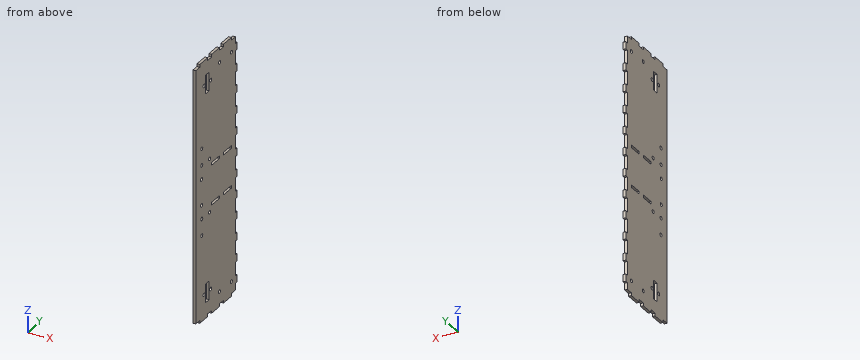
from build123d import *

# Parameters (mm, degrees)
SKETCH1_W               = 279.4
SKETCH1_H               = 76.2
BOSS_EXTRUDE1_DEPTH     = 3
SKETCH3_W               = 3
SKETCH3_H               = 7.8
CUT_EXTRUDE1_DEPTH      = 145.833352512
LPATTERN1_COUNT         = 4
LPATTERN1_PITCH         = 22.8
MIRROR1_COPY_1_SKETCH_W = 3
MIRROR1_COPY_1_SKETCH_H = 7.8
MIRROR1_COPY_1_DEPTH    = 145.833352512
MIRROR1_COPY_2_SKETCH_W = 3
MIRROR1_COPY_2_SKETCH_H = 7.8
MIRROR1_COPY_2_DEPTH    = 145.833352512
MIRROR1_COPY_3_SKETCH_W = 3
MIRROR1_COPY_3_SKETCH_H = 7.8
MIRROR1_COPY_3_DEPTH    = 145.833352512
SKETCH5_W               = 3
SKETCH5_H               = 15
CUT_EXTRUDE3_DEPTH      = 10
SKETCH9_W               = 3
SKETCH9_H               = 7.8
BOSS_EXTRUDE2_DEPTH     = 3
LPATTERN4_COUNT         = 12
LPATTERN4_PITCH         = 22.8
LPATTERN5_COUNT         = 2
LPATTERN5_PITCH         = 22.8
MIRROR2_COPY_1_SKETCH_W = 3
MIRROR2_COPY_1_SKETCH_H = 15
MIRROR2_COPY_1_DEPTH    = 10
F_6_CLEARANCE_HOLE1_D   = 3.7973
CUT_EXTRUDE4_REACH      = 147.651
SKETCH12_W              = 20.2
SKETCH12_H              = 6.7
F_6_CLEARANCE_HOLE2_D   = 3.7973
F_6_CLEARANCE_HOLE3_D   = 3.7973
F_6_CLEARANCE_HOLE4_D   = 3.7973


with BuildPart() as part:
    # Sketch1 → Boss-Extrude1 (new body)
    with BuildSketch(Plane(origin=(0, 0, 0), x_dir=(0, 0, -1), z_dir=(1, 0, 0))):
        Rectangle(SKETCH1_W, SKETCH1_H)
    extrude(amount=-BOSS_EXTRUDE1_DEPTH)

    # Sketch3 → Cut-Extrude1 (cut, through all)
    with BuildSketch(Plane.ZY.offset(3)):
        with Locations((-138.2, 34.2)):
            Rectangle(SKETCH3_W, SKETCH3_H)
    cut_extrude1 = extrude(amount=-CUT_EXTRUDE1_DEPTH, mode=Mode.SUBTRACT)

    # LPattern1: Cut-Extrude1 ×4
    with Locations(*[(0, -i * LPATTERN1_PITCH, 0) for i in range(1, LPATTERN1_COUNT)]):
        add(cut_extrude1, mode=Mode.SUBTRACT)

    # Mirror1: Cut-Extrude1 across plane
    add(cut_extrude1.mirror(Plane.XY), mode=Mode.SUBTRACT)

    # Mirror1 copy 1 sketch → Mirror1 copy 1 (cut, through all)
    with BuildSketch(Plane(origin=(-3, -22.8, 0), x_dir=(0, 0, -1), z_dir=(-1, 0, 0))):
        with Locations((-138.2, -34.2)):
            Rectangle(MIRROR1_COPY_1_SKETCH_W, MIRROR1_COPY_1_SKETCH_H)
    extrude(amount=-MIRROR1_COPY_1_DEPTH, mode=Mode.SUBTRACT)

    # Mirror1 copy 2 sketch → Mirror1 copy 2 (cut, through all)
    with BuildSketch(Plane(origin=(-3, -45.6, 0), x_dir=(0, 0, -1), z_dir=(-1, 0, 0))):
        with Locations((-138.2, -34.2)):
            Rectangle(MIRROR1_COPY_2_SKETCH_W, MIRROR1_COPY_2_SKETCH_H)
    extrude(amount=-MIRROR1_COPY_2_DEPTH, mode=Mode.SUBTRACT)

    # Mirror1 copy 3 sketch → Mirror1 copy 3 (cut, through all)
    with BuildSketch(Plane(origin=(-3, -68.4, 0), x_dir=(0, 0, -1), z_dir=(-1, 0, 0))):
        with Locations((-138.2, -34.2)):
            Rectangle(MIRROR1_COPY_3_SKETCH_W, MIRROR1_COPY_3_SKETCH_H)
    extrude(amount=-MIRROR1_COPY_3_DEPTH, mode=Mode.SUBTRACT)

    # Sketch5 → Cut-Extrude3 (cut)
    with BuildSketch(Plane.ZY.offset(3)):
        with Locations((-21.5, 22.8)):
            Rectangle(SKETCH5_W, SKETCH5_H)
    cut_extrude3 = extrude(amount=-CUT_EXTRUDE3_DEPTH, mode=Mode.SUBTRACT)

    # Sketch9 → Boss-Extrude2 (add)
    with BuildSketch(Plane(origin=(0, 38.1, 0), x_dir=(1, 0, 0), z_dir=(0, 1, 0))):
        with Locations((-1.5, 125.4)):
            Rectangle(SKETCH9_W, SKETCH9_H)
    boss_extrude2 = extrude(amount=BOSS_EXTRUDE2_DEPTH)

    # LPattern4: Boss-Extrude2 ×12
    with Locations(*[(0, 0, i * LPATTERN4_PITCH) for i in range(1, LPATTERN4_COUNT)]):
        add(boss_extrude2)

    # LPattern5: Cut-Extrude3 ×2
    with Locations(*[(0, -i * LPATTERN5_PITCH, 0) for i in range(1, LPATTERN5_COUNT)]):
        add(cut_extrude3, mode=Mode.SUBTRACT)

    # Mirror2: Cut-Extrude3 across plane
    add(cut_extrude3.mirror(Plane.XY), mode=Mode.SUBTRACT)

    # Mirror2 copy 1 sketch → Mirror2 copy 1 (cut)
    with BuildSketch(Plane(origin=(-3, -22.8, 0), x_dir=(0, 0, -1), z_dir=(-1, 0, 0))):
        with Locations((-21.5, -22.8)):
            Rectangle(MIRROR2_COPY_1_SKETCH_W, MIRROR2_COPY_1_SKETCH_H)
    extrude(amount=-MIRROR2_COPY_1_DEPTH, mode=Mode.SUBTRACT)

    # #6 Clearance Hole1 (through all)
    with Locations(Plane(origin=(0, 0, 0), x_dir=(0, 0, -1), z_dir=(1, 0, 0))):
        with Locations((-28.9, -11.55), (-28.9, -26.55), (28.9, -26.55), (28.9, -11.55), (-46.9, -26.55), (46.9, -26.55)):
            Hole(F_6_CLEARANCE_HOLE1_D / 2)

    # Sketch12 → Cut-Extrude4 (cut, up to next)
    with BuildSketch(Plane(origin=(0, 0, 0), x_dir=(0, 0, -1), z_dir=(1, 0, 0)), mode=Mode.PRIVATE) as cut_extrude4_sk1:
        with Locations((-112.7, -15.8)):
            Rectangle(SKETCH12_W, SKETCH12_H)
    cut_extrude4_tool1 = extrude(cut_extrude4_sk1.sketch, amount=-CUT_EXTRUDE4_REACH, mode=Mode.PRIVATE) & part.part
    # Sketch12 → Cut-Extrude4 (cut, up to next)
    with BuildSketch(Plane(origin=(0, 0, 0), x_dir=(0, 0, -1), z_dir=(1, 0, 0)), mode=Mode.PRIVATE) as cut_extrude4_sk2:
        with Locations((112.7, -15.8)):
            Rectangle(SKETCH12_W, SKETCH12_H)
    cut_extrude4_tool2 = extrude(cut_extrude4_sk2.sketch, amount=-CUT_EXTRUDE4_REACH, mode=Mode.PRIVATE) & part.part
    add(cut_extrude4_tool1.solids().sort_by_distance((0, -15.8, 112.7))[0], mode=Mode.SUBTRACT)
    add(cut_extrude4_tool2.solids().sort_by_distance((0, -15.8, -112.7))[0], mode=Mode.SUBTRACT)

    # #6 Clearance Hole2 (through all)
    with Locations(Plane.ZY.offset(3)):
        with Locations((-112.7, -9.45), (-112.7, -22.15), (112.7, -22.15), (112.7, -9.45)):
            Hole(F_6_CLEARANCE_HOLE2_D / 2)

    # #6 Clearance Hole3 (through all)
    with Locations(Plane.ZY.offset(3)):
        with Locations((14, -27.1), (-14, -27.1)):
            Hole(F_6_CLEARANCE_HOLE3_D / 2)

    # #6 Clearance Hole4 (through all)
    with Locations(Plane.ZY.offset(3)):
        with Locations((-123.7, 30.3), (-123.7, 7.5), (123.7, 7.5), (123.7, 30.3)):
            Hole(F_6_CLEARANCE_HOLE4_D / 2)


solid = part.part
Source: CAD feature listing. Evaluate the final solid. Frame: model axes, mm. Coordinates: 2 decimals unless noted, no trailing zeros. Loops run counter-clockwise (first coordinate to the right, second up) from the corner with the lowest first, then second, coordinate; pieces in that order, holes last. Notation, with made-up numbers: (-21, 55) - (26, 55) arc R16 cw to (26, 70) - close; hole circle Ø5 at (39.25, 82). An arc over 180 degrees is marked (long way). One line per item, written item: value. Start each with the question number.
1. Section C-C (x = -1.6). State how many separate pieces and enclosed holes the cut face has, and give its area (3 significant figures).
2. Ray query, L1, parallel to Z at x = -0.2, y = 4.5; L2, parallel to Y at x = -1.8, z = 112.7; L3, parallel to Y at x = -2.25, z = 28.9. Return the intervals inside material, ascending.
3. Section D-D (y = 12). Return the cut outline in (x, z).
4. Section B-B (z = 42). Return the cut outline in (x, y), and give its area (3 significant figures).
5. Contact query for flat-ended pins moving along their axis: P1, Ø0.9, axis at x = -1.5, z = 138.5, coming from the +Y side; P2, Ø0.9, axis at x = -1, y = 39.5, coming from the -Z side; P3, Ø1.5, axis at x = -1, y = 11, coming from the +Z side. Output: stop coordinate, or through.
6. Section A-A (y = -3.5). Return the cut outline in (x, z).
Verdict:
1. separate pieces: 1
1. enclosed holes: 22
1. area: 20,800 mm2
2. L1: z = -139.7 to -23, -20 to 20, 23 to 139.7
2. L2: y = -38.1 to -24.05, -20.25 to -19.15, -12.45 to -11.35, -7.55 to 38.1
2. L3: y = -38.1 to -28.45, -24.65 to -13.45, -9.65 to 38.1
3. outline: (-3, -136.7) - (0, -136.7) - (0, 136.7) - (-3, 136.7) - close
4. outline: (-3, -38.1) - (0, -38.1) - (0, 38.1) - (-3, 38.1) - close
4. area: 229 mm2
5. P1: stops at y = 30.3
5. P2: stops at z = -129.3
5. P3: stops at z = 136.7
6. outline: (-3, -139.7) - (0, -139.7) - (0, -23) - (-3, -23) - close; (-3, -20) - (0, -20) - (0, 20) - (-3, 20) - close; (-3, 23) - (0, 23) - (0, 139.7) - (-3, 139.7) - close
